```python
from build123d import *

# Parameters (mm, degrees)
F0_W     = 381
F0_H     = 88.9
F1_DEPTH = 44.45
F5_W     = 12.7
F5_H     = 6.35
F6_DEPTH = 381.001
F4_W     = 88.9
F4_H     = 88.9
F4_W_2   = 38.1
F4_H_2   = 50.8
F7_REACH = 193.287585695
F8_W     = 88.9
F8_H     = 88.9
F8_W_2   = 38.1
F8_H_2   = 50.8
F9_DEPTH = 38.1


with BuildPart() as f1:
    # F0 (on Right) → F1 (new body, symmetric)
    with BuildSketch(Plane.YZ):
        Rectangle(F0_W, F0_H)
    extrude(amount=F1_DEPTH, both=True)

    # F5 (on face) → F6 (cut, through all)
    with BuildSketch(Plane(origin=(0, 190.5, 0), x_dir=(-1, 0, 0), z_dir=(0, 1, 0))):
        with Locations((38.1, 41.275)):
            Rectangle(F5_W, F5_H)
    extrude(amount=-F6_DEPTH, mode=Mode.SUBTRACT)

    f7_end = Plane(origin=(0, 111.4494145991, 64.3453495198), x_dir=(0, 0.5, -0.8660254038), z_dir=(0, -0.8660254038, -0.5))
    # F4 (on face) → F7 (cut, up to a plane its end follows)
    with BuildSketch(Plane(origin=(0, 190.5, 0), x_dir=(-1, 0, 0), z_dir=(0, 1, 0))):
        Rectangle(F4_W, F4_H)
        Rectangle(F4_W_2, F4_H_2, mode=Mode.SUBTRACT)
    f7_long = extrude(amount=-F7_REACH, mode=Mode.PRIVATE)
    add(split(f7_long, bisect_by=f7_end, keep=Keep.BOTTOM, mode=Mode.PRIVATE), mode=Mode.SUBTRACT)

    # F8 (on face) → F9 (cut)
    with BuildSketch(Plane.XZ.offset(190.5)):
        Rectangle(F8_W, F8_H)
        Rectangle(F8_W_2, F8_H_2, mode=Mode.SUBTRACT)
    extrude(amount=-F9_DEPTH, mode=Mode.SUBTRACT)


solid = f1.part
```
Could you check a few things on this model? Use its own coordinates, in mm. A direction names the side the tool comes from. Give positions to 0.01 mm unless a question says otherwise; leave off trailing zeros. Loops run counter-clockwise (first coordinate to the right, second up) from the corner with the lowest first, then second, coordinate; pieces in that order, holes last. Notation, with made-up numbers: (-31.75, 12) - (-0.75, 12) arc R20 ccw to (-0.75, 17) - close; hole circle Ø4 at (54.5, 56). An arc over 180 degrees is marked (long way). Use one line per item in the form item = value.
1. I want a section at B-B (z = 18). Please give me the cut outline in (x, y), and give its area (3 significant figures).
Response values:
outline = (-44.45, -152.4) - (-19.05, -152.4) - (-19.05, -190.5) - (19.05, -190.5) - (19.05, -152.4) - (44.45, -152.4) - (44.45, 138.21) - (19.05, 138.21) - (19.05, 190.5) - (-19.05, 190.5) - (-19.05, 138.21) - (-44.45, 138.21) - close
area = 29,300 mm²
2. I'm going to push flat-ended pins straight in: pin 1 Ø5 at (y, z) = (149.5, 18) entering from -X; pin 2 Ø5 at (y, z) = (-68.5, 40.5) entering from -X; pin 3 Ø6.5 at (x, y) = (-40.5, 22) entering from +Z; pin 4 Ø19 at (x, y) = (-6.5, -163.5) entering from +Z. Where does each tip first touch, or does it pass through?
Response values:
pin_1 = -19.05
pin_2 = -44.45
pin_3 = 38.1
pin_4 = 25.4
3. I want a section at A-A (x = 6.5). Please give me the cut outline in (y, z).
Response values:
outline = (-190.5, -25.4) - (-152.4, -25.4) - (-152.4, -44.45) - (174.26, -44.45) - (163.26, -25.4) - (190.5, -25.4) - (190.5, 25.4) - (133.93, 25.4) - (122.94, 44.45) - (-152.4, 44.45) - (-152.4, 25.4) - (-190.5, 25.4) - close
4. I want a section at C-C (y = -163). Please give me the cut outline in (x, z).
Response values:
outline = (-19.05, -25.4) - (19.05, -25.4) - (19.05, 25.4) - (-19.05, 25.4) - close
5. On a 3-axis mill with a long thin cutter (end or side, diameter ignored), from which of +Z, -Z, +X, -X, +Y, -Y can I reach the whole of each face in a straight line? I mean faces 1 (the face through (0, -172, -25.4)), 2 (the face through (0, -172, 25.4)), 3 (the face through (19.05, 169, 0)), 4 (the face through (-19.05, -172, 0)). Say none if no direction works.
Response values:
face_1 = -Z, +X, -X, -Y
face_2 = +Z, +X, -X, -Y
face_3 = +Z, +X, +Y
face_4 = +Z, -Z, -X, -Y
6. I want a section at D-D (x = 39.5). Please give me the cut outline in (y, z), and give its area (3 significant figures).
Response values:
outline = (-152.4, -44.45) - (174.26, -44.45) - (122.94, 44.45) - (-152.4, 44.45) - close
area = 26,800 mm²
7. I need wall thicknesses on probe 1 along X at (y, z) = (-122, 40); probe 2 along X at (y, z) = (175, -13); probe 3 along Y at (x, z) = (-40, 28). Which ranges of each line are inside material? Lowest first, please.
Response values:
probe_1 = -31.75 to 44.45
probe_2 = -19.05 to 19.05
probe_3 = -152.4 to 132.43
